```python
from build123d import *

# Parameters (mm, degrees)
EXTRUDE_1_DEPTH          = 1.5
SKETCH_2_R               = 28
EXTRUDE_2_DEPTH          = 3
FILLET_1_R               = 2
SKETCH_3_R               = 1.275
CUT_EXTRUDE_1_DEPTH      = 4
SKETCH_4_R               = 2.025
CUT_EXTRUDE_2_DEPTH      = 4
SKETCH_5_W               = 25
SKETCH_5_H               = 6
CUT_EXTRUDE_3_DEPTH      = 4
FILLET_2_R               = 2
SKETCH_6_R               = 2.025
CUT_EXTRUDE_4_DEPTH      = 10
FILLET_3_R               = 5
SKETCH_7_R               = 2.025
CUT_EXTRUDE_5_DEPTH      = 1
CUT_EXTRUDE_5_DEPTH_BACK = 4
CUT_EXTRUDE_6_DEPTH      = 10
FILLET_4_R               = 3


with BuildPart() as part:
    # 草图1 → 凸台-拉伸1 (new body, symmetric)
    with BuildSketch(Plane.XY):
        Polygon((0, 0), (0, 24), (-7, 30), (-35, 30), (-35, 50), (25, 50), (25, 0), align=None)
    extrude(amount=EXTRUDE_1_DEPTH, both=True)

    # 草图2 → 凸台-拉伸2 (add)
    with BuildSketch(Plane.XY.offset(1.5)):
        with Locations((8.7, 65)):
            Circle(SKETCH_2_R)
    extrude(amount=-EXTRUDE_2_DEPTH)

    # 圆角1
    fillet_1_edges = [part.edges().sort_by_distance(p)[0] for p in [
        (0, 0, 0),
        (0, 24, 0),
        (-7, 30, 0),
        (-35, 30, 0),
        (-35, 50, 0),
        (25, 0, 0),
    ]]
    fillet(fillet_1_edges, radius=FILLET_1_R)

    # 草图3 → 切除-拉伸1 (cut, through all)
    with BuildSketch(Plane.XY.offset(1.5)):
        with Locations((22.135028843, 78.435028843)):
            Circle(SKETCH_3_R)
        with Locations((27.7, 65)):
            Circle(SKETCH_3_R)
        with Locations((22.135028843, 51.564971157)):
            Circle(SKETCH_3_R)
        with Locations((8.7, 46)):
            Circle(SKETCH_3_R)
        with Locations((-4.735028843, 51.564971157)):
            Circle(SKETCH_3_R)
        with Locations((-10.3, 65)):
            Circle(SKETCH_3_R)
        with Locations((-4.735028843, 78.435028843)):
            Circle(SKETCH_3_R)
        with Locations((8.7, 84)):
            Circle(SKETCH_3_R)
    extrude(amount=-CUT_EXTRUDE_1_DEPTH, mode=Mode.SUBTRACT)

    # 草图4 → 切除-拉伸2 (cut, through all)
    with BuildSketch(Plane.XY.offset(1.5)):
        with Locations((12.55, 22)):
            Circle(SKETCH_4_R)
        with Locations((12.55, 12)):
            Circle(SKETCH_4_R)
    extrude(amount=-CUT_EXTRUDE_2_DEPTH, mode=Mode.SUBTRACT)

    # 草图5 → 切除-拉伸3 (cut, through all)
    with BuildSketch(Plane.XY.offset(1.5)):
        with Locations((12.5, 3)):
            Rectangle(SKETCH_5_W, SKETCH_5_H)
    extrude(amount=-CUT_EXTRUDE_3_DEPTH, mode=Mode.SUBTRACT)

    # 圆角2
    fillet_2_edges = [part.edges().sort_by_distance(p)[0] for p in [
        (0, 6, 0),
        (25, 6, 0),
    ]]
    fillet(fillet_2_edges, radius=FILLET_2_R)

    # 草图6 → 切除-拉伸4 (cut)
    with BuildSketch(Plane.XY.offset(1.5)):
        with Locations((-30, 46)):
            Circle(SKETCH_6_R)
        with Locations((-30, 34)):
            Circle(SKETCH_6_R)
    extrude(amount=-CUT_EXTRUDE_4_DEPTH, mode=Mode.SUBTRACT)

    # 圆角3
    fillet_3_edges = [part.edges().sort_by_distance(p)[0] for p in [
        (25, 42.233577356, 0),
        (-14.943180835, 50, 0),
    ]]
    fillet(fillet_3_edges, radius=FILLET_3_R)

    # 草图7 → 切除-拉伸5 (cut, two sides)
    with BuildSketch(Plane.XY.offset(1.5)) as cut_extrude_5_sk:
        with Locations((-21, 46)):
            Circle(SKETCH_7_R)
        with Locations((-21, 34)):
            Circle(SKETCH_7_R)
    extrude(amount=CUT_EXTRUDE_5_DEPTH, mode=Mode.SUBTRACT)
    extrude(cut_extrude_5_sk.sketch, amount=-CUT_EXTRUDE_5_DEPTH_BACK, mode=Mode.SUBTRACT)

    # 草图8 → 切除-拉伸6 (cut)
    with BuildSketch(Plane.XY.offset(1.5)):
        Polygon((8.7, 78.529902504), (-0.867085809, 74.567085809), (-4.829902504, 65), (-0.867085809, 55.432914191), (8.7, 51.470097496), (18.267085809, 55.432914191), (22.229902504, 65), (18.267085809, 74.567085809), align=None)
    extrude(amount=-CUT_EXTRUDE_6_DEPTH, mode=Mode.SUBTRACT)

    # 圆角4
    fillet_4_edges = [part.edges().sort_by_distance(p)[0] for p in [
        (8.7, 78.529902504, 0),
        (18.267085809, 74.567085809, 0),
        (22.229902504, 65, 0),
        (18.267085809, 55.432914191, 0),
        (8.7, 51.470097496, 0),
        (-0.867085809, 55.432914191, 0),
        (-4.829902504, 65, 0),
        (-0.867085809, 74.567085809, 0),
    ]]
    fillet(fillet_4_edges, radius=FILLET_4_R)


solid = part.part
```
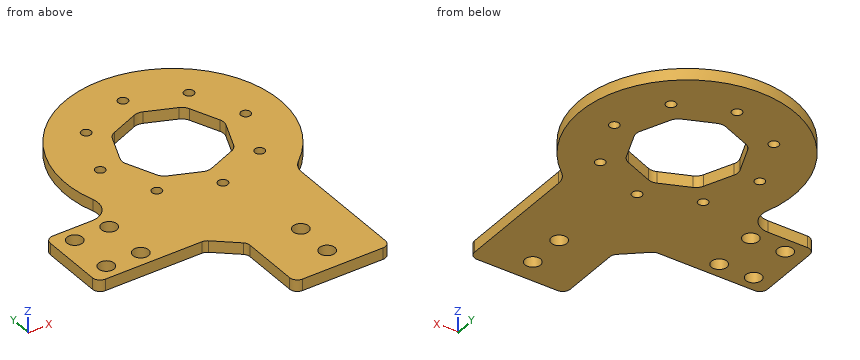
The listing builds one solid part. Answer for the finished solid, in the listing's coordinates (mm). Round coordinates to 2 decimals unless told otherwise and drop trailing zeros. Loops run counter-clockwise (first coordinate to the right, second up) from the corner with the lowest first, then second, coordinate; pieces in that order, holes last.
Q1. Section B-B, the plane x = 6 is taken. Determine the outline of the cut face in (y, z).
Q2. Find the intervals of material crossed by line 1 (Y direction, x = -30, z = -1.3) (3 decimals); line 2 (Y direction, x = 9.5, z = 0.65); line 3 (Y direction, x = -19.5, z = 0.7), in increasing order.
Q3. Section D-D, the plane y = 65 is taken. Determine the outline of the cut face in (x, z) (3 decimals).
Q4. Section A-A, the plane y = 34 is taken. Determine the outline of the cut face in (x, z) (3 decimals).
Q5. Section C-C, the plane y = 12 is taken. Determine the outline of the cut face in (x, z) (3 decimals), then the cut area to 4 significant figures.
Q6. Given pin 1 Ø5.5 at (x, y) = (-30, 34) entering from +Z; pin 2 Ø1.5 at (y, z) = (18, 0.5) entering from -X; pin 3 Ø1.5 at (x, z) = (-11.5, 0.5) entering from -Y, each flat-ended and moving along its own axis, determine where each tip first touches the part or whether it passes through.
Completed:
1. outline: (6, -1.5) - (52.59, -1.5) - (52.59, 1.5) - (6, 1.5) - close; (77.41, -1.5) - (92.87, -1.5) - (92.87, 1.5) - (77.41, 1.5) - close
2. line 1: y = 30 to 31.975, 36.025 to 43.975, 48.025 to 50
2. line 2: y = 6 to 45.01, 46.99 to 51.83, 78.17 to 83.01, 84.99 to 92.99
2. line 3: y = 30 to 32.64, 35.36 to 44.64, 47.36 to 51.2
3. outline: (-19.3, -1.5) - (-11.575, -1.5) - (-11.575, 1.5) - (-19.3, 1.5) - close; (-9.025, -1.5) - (-4.583, -1.5) - (-4.583, 1.5) - (-9.025, 1.5) - close; (21.983, -1.5) - (26.425, -1.5) - (26.425, 1.5) - (21.983, 1.5) - close; (28.975, -1.5) - (36.7, -1.5) - (36.7, 1.5) - (28.975, 1.5) - close
4. outline: (-35, -1.5) - (-32.025, -1.5) - (-32.025, 1.5) - (-35, 1.5) - close; (-27.975, -1.5) - (-23.025, -1.5) - (-23.025, 1.5) - (-27.975, 1.5) - close; (-18.975, -1.5) - (25, -1.5) - (25, 1.5) - (-18.975, 1.5) - close
5. outline: (0, -1.5) - (10.525, -1.5) - (10.525, 1.5) - (0, 1.5) - close; (14.575, -1.5) - (25, -1.5) - (25, 1.5) - (14.575, 1.5) - close
5. area: 62.85 mm2
6. pin 1: stops at z = 1.5
6. pin 2: stops at x = 0
6. pin 3: stops at y = 30
